Can you work these out from the drawing? Everything is in mm from the part's minimum corner. Round coordinates to 2 decimals unless told otherwise and drop trailing zeros. Write each loop counter-clockwise with the first axis right and the second up, starting at its lowest first coordinate (ties: lowest second). Pieces come first, ordered by that corner, then holes. Notation, with made-up numbers: (21, 5.5) - (57, 5.5) arc R15 cw to (57, 24.5) - close; hole circle Ø5 at (27, -28.75). An arc over 180 degrees is marked (long way). Write each question's results on one line, items separated by ' | '. Start each with the question number.
(1) Imagine slicing it at D-D on x = 52. Write out the boundary of the cut face in (y, z).
(2) Please list where these lines run through material, in increasing order: line 1 (X direction, y = 59.5, z = 2.05); line 2 (Y direction, x = 31.5, z = 2.1); line 3 (Y direction, x = 52, z = 2.4). Write a range as [from, to].
(3) Imagine slicing it at A-A on y = 19. Write out the boundary of the cut face in (x, z).
(4) For P1, Ø1.5, axis at x = 4, z = 1, coming from the -Y side; P2, Ø0.9, axis at y = 21.5, z = 1.5, coming from the -X side, each with a flat end and sliding along its axis, tell me the tip position at first contact or that it passes through.
(5) Imagine slicing it at B-B on x = 40.5. Write out the boundary of the cut face in (y, z), then the cut area to 3 significant figures.
(6) Imagine slicing it at C-C on z = 1.8. State how many separate pieces and enclosed holes the cut face has, then the cut area to 3 significant figures.
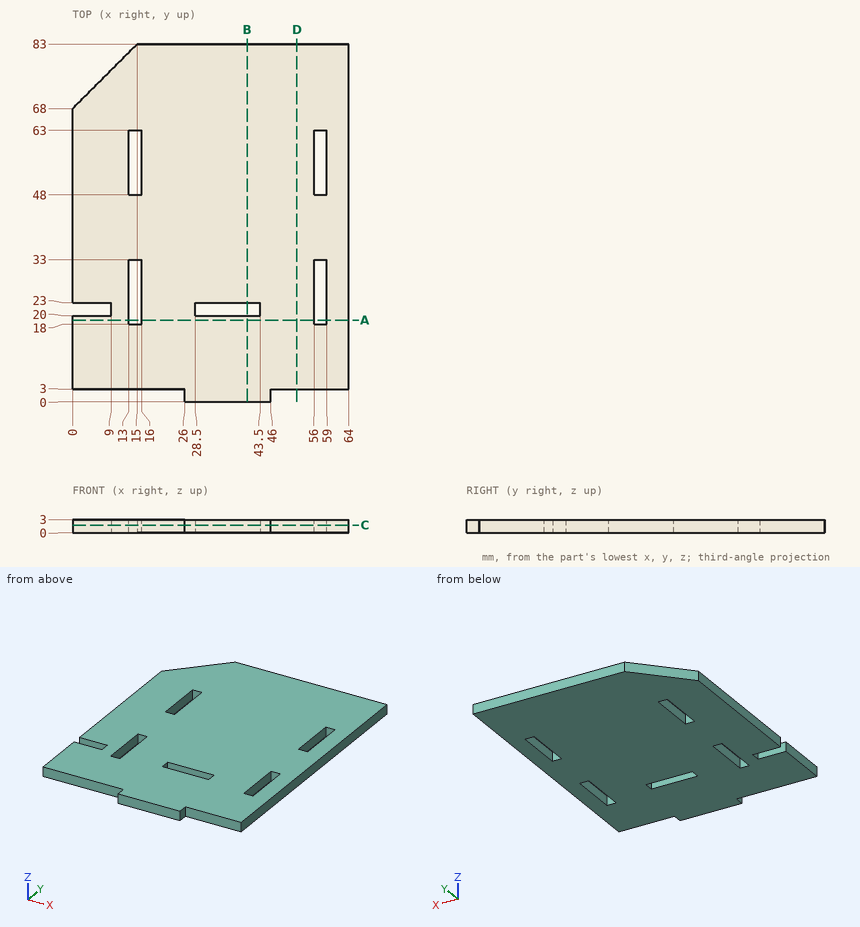
Response:
1) outline: (3, 0) - (83, 0) - (83, 3) - (3, 3) - close
2) line 1: [0, 13], [16, 56], [59, 64] | line 2: [0, 20], [23, 83] | line 3: [3, 83]
3) outline: (0, 0) - (13, 0) - (13, 3) - (0, 3) - close; (16, 0) - (56, 0) - (56, 3) - (16, 3) - close; (59, 0) - (64, 0) - (64, 3) - (59, 3) - close
4) P1: y = 3 | P2: x = 9
5) outline: (0, 0) - (20, 0) - (20, 3) - (0, 3) - close; (23, 0) - (83, 0) - (83, 3) - (23, 3) - close | area: 240 mm²
6) separate pieces: 1 | enclosed holes: 5 | area: 4,820 mm²
